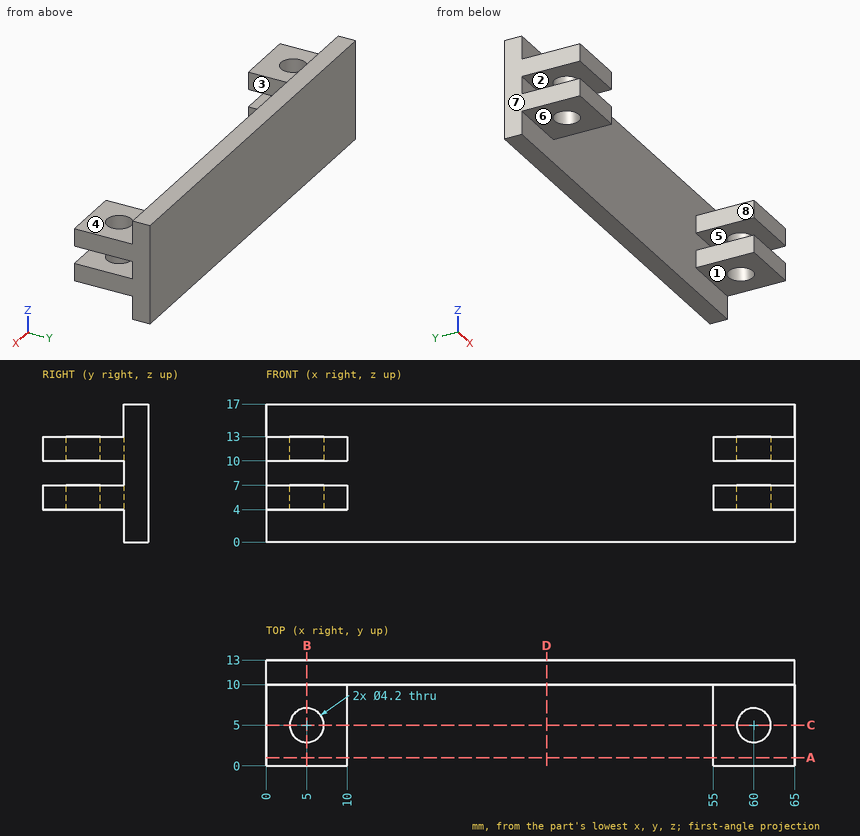
Design review of the part shown in the three views and the two pictorial views. Dimensions are in mm from the part's minimum x, y and z. A direction names the side the tool comes from. Round coordinates to 2 decimals unless told otherwise and drop trailing zeros. Order: outer loops, then holes, each group sorted by start corner. A loop starts at its lowest first (then second) coordinate and runs counter-clockwise, first axis right, second up. Notation, with made-up numbers: M 46.5,3.25 L 92.5,3.25 A17 cw 92.5,11.25 Z; hole C 39.25,-12.5 d4. An arc over 180 degrees is marked long. Put each result on its own line as item: value.
Q1. Consider section D-D (x = 34.5). State the section outline as (y, z) points, and give its area (3 significant figures).
Reported:
outline: M 10,0 L 13,0 L 13,17 L 10,17 Z
area: 51.0 mm²
Q2. Consider section A-A (y = 1). State the section outline as (x, z) points.
Reported:
outline: M 0,4 L 10,4 L 10,7 L 0,7 Z; M 0,10 L 10,10 L 10,13 L 0,13 Z; M 55,4 L 65,4 L 65,7 L 55,7 Z; M 55,10 L 65,10 L 65,13 L 55,13 Z
Q3. Consider section B-B (x = 5). State the section outline as (y, z) points, and give its area (3 significant figures).
Reported:
outline: M 0,4 L 2.9,4 L 2.9,7 L 0,7 Z; M 0,10 L 2.9,10 L 2.9,13 L 0,13 Z; M 7.1,4 L 10,4 L 10,0 L 13,0 L 13,17 L 10,17 L 10,13 L 7.1,13 L 7.1,10 L 10,10 L 10,7 L 7.1,7 Z
area: 85.8 mm²
Q4. Machinability: for the marked faces 4, 5, 6, 7 and 8, which of the approach directions +Z, -Z, +X, -X, +Y, -Y give a long, thin tool a straight path to every point of the face, cutting with its end or side? Answer none if there is none.
Reported:
face 4: +Z, +X, -X, -Y
face 5: +X, -X, -Y
face 6: -Z, +X, -X, -Y
face 7: +Z, -Z, -X, +Y, -Y
face 8: +Z, -Z, -Y
Q5. To check wall thickness, follow line 1 (Z direction, x = 9.5, y = 1); line 2 (Y direction, x = 5, z = 10.85); line 3 (X direction, y = 5.25, z = 11). State the ranges of each line that lie inside material, in increasing order.
Reported:
line 1: 4 to 7, 10 to 13
line 2: 0 to 2.9, 7.1 to 13
line 3: 0 to 2.91, 7.09 to 10, 55 to 57.91, 62.09 to 65
Q6. Draft analysis for pull direction Z (two halves, no side actions). For the marked faces 1, 2 and 3, state which applies: released by +Z, released by -Z, zero draft, split by the parting line, or undercut.
Reported:
face 1: released by -Z
face 2: undercut
face 3: zero draft
Q7. Consider section C-C (y = 5). State how many separate pieces and enclosed holes the cut face has, and give its area (3 significant figures).
Reported:
separate pieces: 8
enclosed holes: 0
area: 69.6 mm²
Q8. Insertion check: pin 1 Ø5 at (x, y) = (58, 7) entering from -Z; pin 2 Ø5 at (x, y) = (6.5, 5) entering from +Z; pin 3 Ø8.5 at (x, z) = (45.5, 8) entering from -Y; pin 4 Ø3.5 at (x, y) = (60, 5) entering from +Z (3 decimals). Each pin has a flat end and moves straight along its axis. Give the tip position at first contact, or say it passes through.
Reported:
pin 1: z = 4
pin 2: z = 13
pin 3: y = 10
pin 4: through
